from build123d import *

# Parameters (mm, degrees)
SKETCH1_R           = 51
SKETCH1_R_2         = 39
SKETCH1_R_3         = 1.5
BOSS_EXTRUDE1_DEPTH = 5
FILLET1_R           = 3
SKETCH2_R           = 2.75
CUT_EXTRUDE1_DEPTH  = 3
SKETCH3_R           = 41.5
SKETCH3_R_2         = 39
BOSS_EXTRUDE2_DEPTH = 2


with BuildPart() as part:
    # Sketch1 → Boss-Extrude1 (new body)
    with BuildSketch(Plane(origin=(0, 0, 0), x_dir=(1, 0, 0), z_dir=(0, 1, 0))):
        Circle(SKETCH1_R)
        Circle(SKETCH1_R_2, mode=Mode.SUBTRACT)
        with Locations((45.25, 0)):
            Circle(SKETCH1_R_3, mode=Mode.SUBTRACT)
        with Locations((42.521091091, -15.476411485)):
            Circle(SKETCH1_R_3, mode=Mode.SUBTRACT)
        with Locations((34.663511051, -29.086139338)):
            Circle(SKETCH1_R_3, mode=Mode.SUBTRACT)
        with Locations((22.625, -39.187649521)):
            Circle(SKETCH1_R_3, mode=Mode.SUBTRACT)
        with Locations((7.857580039, -44.562550824)):
            Circle(SKETCH1_R_3, mode=Mode.SUBTRACT)
        with Locations((-7.857580039, -44.562550824)):
            Circle(SKETCH1_R_3, mode=Mode.SUBTRACT)
        with Locations((-22.625, -39.187649521)):
            Circle(SKETCH1_R_3, mode=Mode.SUBTRACT)
        with Locations((-34.663511051, -29.086139338)):
            Circle(SKETCH1_R_3, mode=Mode.SUBTRACT)
        with Locations((-42.521091091, -15.476411485)):
            Circle(SKETCH1_R_3, mode=Mode.SUBTRACT)
        with Locations((-45.25, 0)):
            Circle(SKETCH1_R_3, mode=Mode.SUBTRACT)
        with Locations((-42.521091091, 15.476411485)):
            Circle(SKETCH1_R_3, mode=Mode.SUBTRACT)
        with Locations((-34.663511051, 29.086139338)):
            Circle(SKETCH1_R_3, mode=Mode.SUBTRACT)
        with Locations((-22.625, 39.187649521)):
            Circle(SKETCH1_R_3, mode=Mode.SUBTRACT)
        with Locations((-7.857580039, 44.562550824)):
            Circle(SKETCH1_R_3, mode=Mode.SUBTRACT)
        with Locations((7.857580039, 44.562550824)):
            Circle(SKETCH1_R_3, mode=Mode.SUBTRACT)
        with Locations((22.625, 39.187649521)):
            Circle(SKETCH1_R_3, mode=Mode.SUBTRACT)
        with Locations((34.663511051, 29.086139338)):
            Circle(SKETCH1_R_3, mode=Mode.SUBTRACT)
        with Locations((42.521091091, 15.476411485)):
            Circle(SKETCH1_R_3, mode=Mode.SUBTRACT)
    extrude(amount=BOSS_EXTRUDE1_DEPTH)

    # Fillet1
    fillet1_edges = [part.edges().sort_by_distance(p)[0] for p in [
        (-51, 5, 0),
    ]]
    fillet(fillet1_edges, radius=FILLET1_R)

    # Sketch2 → Cut-Extrude1 (cut)
    with BuildSketch(Plane(origin=(0, 5, 0), x_dir=(1, 0, 0), z_dir=(0, 1, 0))):
        with Locations((45.25, 0)):
            Circle(SKETCH2_R)
        with Locations((42.521091091, -15.476411485)):
            Circle(SKETCH2_R)
        with Locations((34.663511051, -29.086139338)):
            Circle(SKETCH2_R)
        with Locations((22.625, -39.187649521)):
            Circle(SKETCH2_R)
        with Locations((7.857580039, -44.562550824)):
            Circle(SKETCH2_R)
        with Locations((-7.857580039, -44.562550824)):
            Circle(SKETCH2_R)
        with Locations((-22.625, -39.187649521)):
            Circle(SKETCH2_R)
        with Locations((-34.663511051, -29.086139338)):
            Circle(SKETCH2_R)
        with Locations((-42.521091091, -15.476411485)):
            Circle(SKETCH2_R)
        with Locations((-45.25, 0)):
            Circle(SKETCH2_R)
        with Locations((-42.521091091, 15.476411485)):
            Circle(SKETCH2_R)
        with Locations((-34.663511051, 29.086139338)):
            Circle(SKETCH2_R)
        with Locations((-22.625, 39.187649521)):
            Circle(SKETCH2_R)
        with Locations((-7.857580039, 44.562550824)):
            Circle(SKETCH2_R)
        with Locations((7.857580039, 44.562550824)):
            Circle(SKETCH2_R)
        with Locations((22.625, 39.187649521)):
            Circle(SKETCH2_R)
        with Locations((34.663511051, 29.086139338)):
            Circle(SKETCH2_R)
        with Locations((42.521091091, 15.476411485)):
            Circle(SKETCH2_R)
    extrude(amount=-CUT_EXTRUDE1_DEPTH, mode=Mode.SUBTRACT)

    # Sketch3 → Boss-Extrude2 (add)
    with BuildSketch(Plane.XZ):
        Circle(SKETCH3_R)
        Circle(SKETCH3_R_2, mode=Mode.SUBTRACT)
    extrude(amount=BOSS_EXTRUDE2_DEPTH)


solid = part.part
Verification items for the finished model (mm, model axes). A direction names the side the tool comes from. Give positions to 0.01 mm unless a question says otherwise; leave off trailing zeros. Loops run counter-clockwise (first coordinate to the right, second up) from the corner with the lowest first, then second, coordinate; pieces in that order, holes last.
1) Thickness scan on line 1 along Z through (x, y) = (-35.5, 0.25); line 2 along Z through (x, y) = (36, 4.25); line 3 along X through (y, z) = (2.5, 30.5). Record the ranges inside material, lowest first.
2) Set-up check for faces 1 (the cylindrical face through (43.75, 0.99, -0.07)), 2 (the cylindrical face through (36.142, 3.521, -31.405)): record each of +Z, -Z, +X, -X, +Y, -Y from which the full face is reachable in a straight line by a thin tool's end or side.
3) Sectioned sample at A-A, the plane x = 0. Enter the section's corners in (y, z), then the cut area to 3 significant figures.
4) Sectioned sample at B-B, the plane y = 3.25. Count the separate pieces of the cut face and the enclosed holes in it, then the cut area to 3 significant figures.
5) Depth check by flat-ended pin: pin 1 Ø4 at (x, z) = (42.52, 15.48) entering from -Y; pin 2 Ø2.5 at (x, z) = (34.66, 29.09) entering from +Y; pin 3 Ø3 at (x, z) = (7.5, -44) entering from +Y; pin 4 Ø1.5 at (y, z) = (-0.5, 13.5) entering from -X. Enter the tip coordinate at first touch or a pass-through.
Answers:
1. line 1: z = -36.62 to -30.33, -27.84 to -16.15, 16.15 to 27.84, 30.33 to 36.62
1. line 2: z = -34.68 to -31.49, -26.68 to -15, 15 to 26.68, 31.49 to 34.68
1. line 3: x = -40.82 to -37.02, -32.3 to -24.31, 24.31 to 32.3, 37.02 to 40.82
2. face 1: +Y, -Y
2. face 2: +Y
3. outline: (-2, -41.5) - (0, -41.5) - (0, -51) - (2, -51) arc R3 ccw to (5, -48) - (5, -39) - (-2, -39) - close; (-2, 39) - (5, 39) - (5, 48) arc R3 ccw to (2, 51) - (0, 51) - (0, 41.5) - (-2, 41.5) - close
3. area: 126 mm2
4. separate pieces: 1
4. enclosed holes: 19
4. area: 2,880 mm2
5. pin 1: stops at y = 0
5. pin 2: passes through
5. pin 3: stops at y = 2
5. pin 4: stops at x = -49.33
